```python
from build123d import *

# Parameters (mm, degrees)
F0_R     = 1.5930303601
F1_DEPTH = 4
F0_R_2   = 1.8103813353
F0_W     = 18
F0_H     = 12
F2_DEPTH = 20
F3_R     = 3.5
F4_DEPTH = 25
F5_R     = 1
F6_DEPTH = 5


with BuildPart() as f1:
    # F0 (on Top) → F1 (new body)
    with BuildSketch(Plane.XY):
        with BuildLine():
            ThreePointArc((0, 6), (1.7573593129, 1.7573593129), (6, 0))
            Line((6, 0), (12, 0))
            Line((12, 0), (12, 12))
            Line((12, 12), (6, 12))
            ThreePointArc((6, 12), (1.7573593129, 10.2426406871), (0, 6))
        make_face()
        with Locations((6, 6)):
            Circle(F0_R, mode=Mode.SUBTRACT)
    extrude(amount=F1_DEPTH)



with BuildPart() as f1b:
    # F0 (on Top) → F1, piece 2 (new body)
    with BuildSketch(Plane.XY):
        with BuildLine():
            Line((30, 12), (30, 0))
            Line((30, 0), (36, 0))
            ThreePointArc((36, 0), (40.2426406871, 1.7573593129), (42, 6))
            ThreePointArc((42, 6), (40.2426406871, 10.2426406871), (36, 12))
            Line((36, 12), (30, 12))
        make_face()
        with Locations((36, 6)):
            Circle(F0_R_2, mode=Mode.SUBTRACT)
    extrude(amount=F1_DEPTH)


with BuildPart() as f1_1:
    add(f1.part)

    add(f1b.part)  # F2 merges F1b
    # F0 (on Top) → F2 (join)
    with BuildSketch(Plane.XY):
        with Locations((21, 6)):
            Rectangle(F0_W, F0_H)
    extrude(amount=F2_DEPTH)

    # F3 (on face) → F4 (cut)
    with BuildSketch(Plane(origin=(12, 0, 0), x_dir=(0, -1, 0), z_dir=(-1, 0, 0))):
        with Locations((-6, 14)):
            Circle(F3_R)
    extrude(amount=-F4_DEPTH, mode=Mode.SUBTRACT)

    # F5 (on face) → F6 (cut)
    with BuildSketch(Plane.XY.offset(20)):
        with Locations((17, 6)):
            Circle(F5_R)
        with Locations((25, 6)):
            Circle(F5_R)
    extrude(amount=-F6_DEPTH, mode=Mode.SUBTRACT)


solid = f1_1.part
```
Design review of the part built by this model. Coordinates are the model's own, in mm. A direction names the side the tool comes from. Round coordinates to 2 decimals unless told otherwise and drop trailing zeros. Order: outer loops, then holes, each group sorted by start corner. A loop starts at its lowest first (then second) coordinate and runs counter-clockwise, first axis right, second up. Notation, with made-up numbers: M 79,-26.75 L 128,-26.75 A16 ccw 128,-18.75 Z; hole C -1,29.25 d3. An arc over 180 degrees is marked long. Put each result on its own line as item: value.
Q1. To check wall thickness, follow line 1 (Y direction, x = 36, z = 2.1); line 2 (X direction, y = 6, z = 18.85); line 3 (Y direction, x = 17, z = 19.35). State the ranges of each line that lie inside material, in increasing order.
Reported:
line 1: 0 to 4.19, 7.81 to 12
line 2: 12 to 16, 18 to 24, 26 to 30
line 3: 0 to 5, 7 to 12
Q2. Consider section B-B (y = 9). State the section outline as (x, z) points.
Reported:
outline: M 0.8,0 L 41.2,0 L 41.2,4 L 30,4 L 30,12.2 L 12,12.2 L 12,4 L 0.8,4 Z; M 12,15.8 L 30,15.8 L 30,20 L 12,20 Z
Q3. Consider section C-C (x = 17). State the section outline as (y, z) points.
Reported:
outline: M 0,0 L 12,0 L 12,20 L 7,20 L 7,17.35 A3.5 cw long 5,17.35 L 5,20 L 0,20 Z
Q4. Insertion check: pin 1 Ø1 at (y, z) = (5.5, 3) entering from +X; pin 2 Ø6 at (y, z) = (3, 14.5) entering from -X; pin 3 Ø3 at (y, z) = (10.5, 9.5) entering from +X. Each pin has a flat end and moves straight along its axis. Give the tip position at first contact, or say it passes through.
Reported:
pin 1: x = 42
pin 2: x = 12
pin 3: x = 30
Q5. Consider section D-D (z = 18). State the section outline as (x, y) points.
Reported:
outline: M 12,0 L 30,0 L 30,12 L 12,12 Z; hole C 17,6 d2; hole C 25,6 d2
Q6. Draft analysis for pull direction X (two halves, no side actions). For faces 4 (the face through (26, 6, 19)), 5 (the face through (12, 6, 10)), 6 (the face through (20.874, 6.759, 10.583)), state which applies: released by +X, released by -X, zero draft, split by the parting line, or undercut.
Reported:
face 4: undercut
face 5: released by -X
face 6: zero draft
Q7. Consider section A-A (z = 14). State the section outline as (x, y) points.
Reported:
outline: M 12,0 L 30,0 L 30,2.5 L 12,2.5 Z; M 12,9.5 L 30,9.5 L 30,12 L 12,12 Z
Q8. Machinability: for faces 1 (the face through (18, 6, 19)), 2 (the face through (34.6, 7.4, 4)), 3 (the face through (7.25, 4.75, 4)), which of the approach directions +Z, -Z, +X, -X, +Y, -Y give a long, thin tool a straight path to every point of the face, cutting with its end or side? Answer none if there is none.
Reported:
face 1: +Z
face 2: +Z, +X, +Y, -Y
face 3: +Z, -X, +Y, -Y
